```python
from build123d import *

# Parameters (mm, degrees)
SKETCH1_W               = 5
SKETCH1_H               = 20
BOSS_EXTRUDE1_DEPTH     = 88.5
CUT_EXTRUDE2_DEPTH      = 35
CUT_EXTRUDE2_DEPTH_BACK = 35
SKETCH5_R               = 35.5
SKETCH2_W               = 5
SKETCH2_H               = 20
CUT_EXTRUDE3_DEPTH      = 13
SKETCH8_W               = 39.75
SKETCH8_H               = 20
CUT_EXTRUDE4_DEPTH      = 13


with BuildPart() as part:
    # Sketch1 → Boss-Extrude1 (new body)
    with BuildSketch(Plane.XY):
        with Locations((-2.5, 10)):
            Rectangle(SKETCH1_W, SKETCH1_H)
    extrude(amount=BOSS_EXTRUDE1_DEPTH)

    # Sketch5 → Cut-Extrude2 (cut, two sides: drawn at the far end of the back side and taken through both)
    with BuildSketch(Plane(origin=(0, 0, 0), x_dir=(0, 0, -1), z_dir=(1, 0, 0)).offset(-CUT_EXTRUDE2_DEPTH_BACK)):
        with Locations((-42.25, 53)):
            Circle(SKETCH5_R)
    extrude(amount=CUT_EXTRUDE2_DEPTH + CUT_EXTRUDE2_DEPTH_BACK, mode=Mode.SUBTRACT)

    # Sketch2 → Cut-Extrude3 (cut)
    with BuildSketch(Plane.ZY.offset(5)):
        with Locations((42.25, 10)):
            Rectangle(SKETCH2_W, SKETCH2_H)
    extrude(amount=-CUT_EXTRUDE3_DEPTH, mode=Mode.SUBTRACT)


with BuildPart() as cut_extrude3_piece_1:
    # of the separate pieces the step leaves, piece 1, a body of its own (cut_extrude3_pieces)
    add(part.part.solids().sort_by_distance((0, 0, 44.75))[0])


with BuildPart() as cut_extrude3_piece_2:
    # of the separate pieces the step leaves, piece 2, a body of its own (cut_extrude3_pieces)
    add(part.part.solids().sort_by_distance((-5, 20, 0))[0])

    # Sketch8 → Cut-Extrude4 (cut)
    with BuildSketch(Plane.ZY.offset(5)):
        with Locations((19.875, 10)):
            Rectangle(SKETCH8_W, SKETCH8_H)
    extrude(amount=-CUT_EXTRUDE4_DEPTH, mode=Mode.SUBTRACT)


solid = cut_extrude3_piece_1.part
```
Here's how the part is built. I have some questions about the finished solid (model axes, mm). Round coordinates to 2 decimals unless told otherwise and drop trailing zeros. Order: outer loops, then holes, each group sorted by start corner. A loop starts at its lowest first (then second) coordinate and runs counter-clockwise, first axis right, second up. Notation, with made-up numbers: M -18,57 L 7,57 A11 cw 7,66 Z; hole C 35.25,1.25 d5. An arc over 180 degrees is marked long. Answer in a Markdown table with one row per item.
Item 1: If I drill on L1, parallel to Y at x = -0.3, z = 51.5; L2, parallel to Y at x = -0.2, z = 49, over which ranges is the centre line in solid material (lowest first)? Write a range as from..to.
A:
| item | result |
|---|---|
| L1 | y = 0..18.73 |
| L2 | y = 0..18.15 |
Item 2: Thinking about a two-plate mould opening in X: for faces 1 (the face through (-3, 0, 66)), 2 (the face through (0, 10, 66)), 3 (the face through (-5, 10, 66)), which applies, +X half, -X half, draft (parallel to the pull), parting line (faces both ways), or undercut?
A:
| item | result |
|---|---|
| face 1 | draft |
| face 2 | +X half |
| face 3 | -X half |
Item 3: Imagine slicing it at B-B, the plane y = 18. Write out the boundary of the cut face in (x, z), and give its area (3 significant figures).
A:
| item | result |
|---|---|
| outline | M -5,48.19 L 0,48.19 L 0,88.5 L -5,88.5 Z |
| area | 202 mm2 |
Item 4: Imagine slicing it at A-A, the plane x = -3.9. Write out the boundary of the cut face in (y, z).
A:
| item | result |
|---|---|
| outline | M 0,44.75 L 17.59,44.75 A35.5 cw 20,55.34 L 20,88.5 L 0,88.5 Z |
